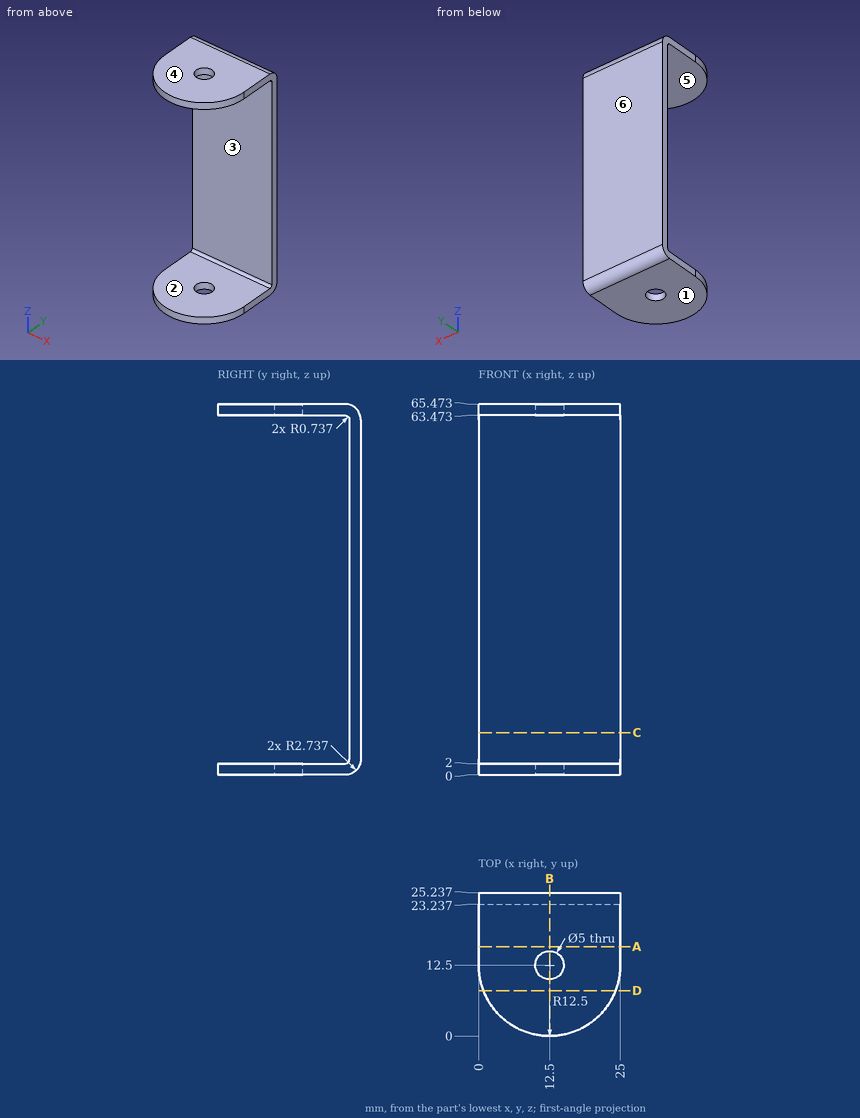
Geometry: see drawing. Coordinates: mm, zero at the bounding-box minimum. A direction names the side the tool comes from. Coordinates: 2 decimals unless noted, no trailing zeros. Order: outer loops, then holes, each group sorted by start corner. A loop starts at its lowest first (then second) coordinate and runs counter-clockwise, first axis right, second up. Notation, with made-up numbers: M 34,2 L 88,2 A20 cw 88,31 Z; hole C 68,-3 d5. An arc over 180 degrees is marked long. Answer in a Markdown table with one row per item. Add a question column.
Q1. Contact query for flat-ended pins moving along their axis: P1, Ø7.5, axis at x = 17, z = 32, coming from the -Y side; P2, Ø12, axis at y = 17, z = 32.5, coming from the -X side. Output: stop coordinate, or through.
Q2. Section query D-D on y = 8. Return the cut outline in (x, z).
Q3. Line query: L1, parallel to Z at x = 10, y = 16.75; L2, parallel to X at y = 12.5, z = 63.95; L3, parallel to Y at x = 8.25, z = 57.5. Output: solid intervals per line, ascending.
Q4. Mould query, pull axis Z, two halves, no side actions, for the marked faces 1, 2, 3 and 4. Classes: released by +Z, released by -Z, zero draft, split by the parting line, or undercut.
Q5. Reachability of the marked faces 5 and 6 from +Z, -Z, +X, -X, +Y, -Y: full face, straight path, thin tool, end or side. Return the list, or none.
Q6. Section query C-C on z = 7.5. Return the cut outline in (x, y), and give its area (3 significant figures).
Q7. Section query A-A on y = 15.75. Return the cut outline in (x, z).
Q8. Section query B-B on x = 12.5. Return the cut outline in (y, z), and give its area (3 significant figures).
Completed:
| question | item | result |
|---|---|---|
| 1 | P1 | stops at y = 23.24 |
| 1 | P2 | passes through |
| 2 | outline | M 0.84,0 L 24.16,0 L 24.16,2 L 0.84,2 Z; M 0.84,63.47 L 24.16,63.47 L 24.16,65.47 L 0.84,65.47 Z |
| 3 | L1 | z = 0 to 2, 63.47 to 65.47 |
| 3 | L2 | x = 0 to 10, 15 to 25 |
| 3 | L3 | y = 23.24 to 25.24 |
| 4 | face 1 | released by -Z |
| 4 | face 2 | undercut |
| 4 | face 3 | undercut |
| 4 | face 4 | released by +Z |
| 5 | face 5 | +X, -X, -Y |
| 5 | face 6 | +Z, -Z, +X, -X, +Y |
| 6 | outline | M 0,23.24 L 25,23.24 L 25,25.24 L 0,25.24 Z |
| 6 | area | 50.0 mm2 |
| 7 | outline | M 0,0 L 25,0 L 25,2 L 0,2 Z; M 0,63.47 L 25,63.47 L 25,65.47 L 0,65.47 Z |
| 8 | outline | M 0,0 L 10,0 L 10,2 L 0,2 Z; M 0,63.47 L 10,63.47 L 10,65.47 L 0,65.47 Z; M 15,0 L 22.5,0 A2.74 ccw 25.24,2.74 L 25.24,62.74 A2.74 ccw 22.5,65.47 L 15,65.47 L 15,63.47 L 22.5,63.47 A0.74 cw 23.24,62.74 L 23.24,2.74 A0.74 cw 22.5,2 L 15,2 Z |
| 8 | area | 201 mm2 |
